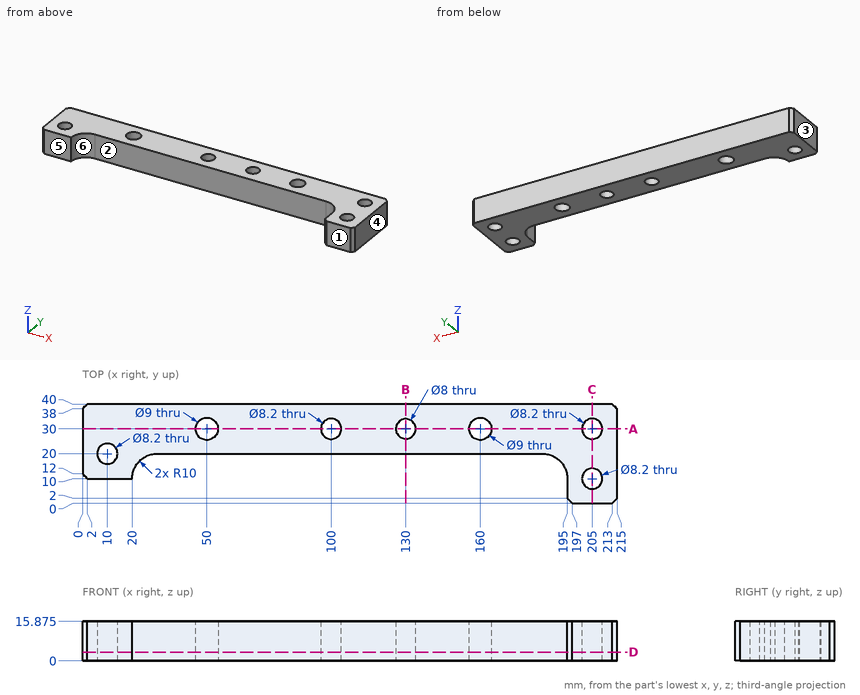
Study the drawing (mm; zero at the part's minimum x, y, z) and answer. A direction names the side the tool comes from. Coordinates: 2 decimals unless noted, no trailing zeros. Write each loop counter-clockwise with the first axis right and the second up, starting at its lowest first coordinate (ties: lowest second). Pieces come first, ordered by that corner, then holes. Notation, with made-up numbers: M -2.5,27.5 L 47.5,27.5 A18 ccw 47.5,33.5 Z; hole C 12.25,33.25 d11. An arc over 180 degrees is marked long. Use a Markdown table: item, result. Add a question column.
1. For a pull along X with two mould halves and no side action, classify the marked faces 3, 4, 5 and 6 as +X half, -X half, draft (parallel to the pull), parting line (faces both ways), or undercut.
2. Section D-D (z = 3.5) is taken. Count the separate pieces of the cut face and the enclosed holes in it, plus the area to 3 significant figures.
3. Section B-B (x = 130) is taken. Give the vertices of the cut face in (y, z) (3 decimals), plus the area to 4 significant figures.
4. Which of the six approach directions +Z, -Z, +X, -X, +Y, -Y give full straight-line access (tool end or side, diameter ignored) to the marked faces 1 and 2?
5. Straight lines are drawn through the part: line 1 along Y through (x, z) = (205, 6.5); line 2 along Y through (x, z) = (10, 6); line 3 along X through (y, z) = (29.5, 12). For each, find the intervals that lie inside material, in ascending order. Write a range as [from, to].
6. Section C-C (x = 205) is taken. Give the vertices of the cut face in (y, z) (3 decimals), plus the area to 3 significant figures.
7. Given P1, Ø8, axis at x = 50, y = 30, coming from the +Z side; P2, Ø2.5, axis at y = 5.5, z = 9, coming from the -X side; P3, Ø8, axis at x = 12, z = 7, coming from the -Y side, each flat-ended and moving along its own axis, determine where each tip first touches the part or whether it passes through.
8. Section A-A (y = 30) is taken. Give the vertices of the cut face in (x, z) (3 decimals).
Data:
| question | item | result |
|---|---|---|
| 1 | face 3 | -X half |
| 1 | face 4 | +X half |
| 1 | face 5 | draft |
| 1 | face 6 | undercut |
| 2 | separate pieces | 1 |
| 2 | enclosed holes | 7 |
| 2 | area | 4,540 mm2 |
| 3 | outline | M 20,0 L 26,0 L 26,15.875 L 20,15.875 Z; M 34,0 L 40,0 L 40,15.875 L 34,15.875 Z |
| 3 | area | 190.5 mm2 |
| 4 | face 1 | +Z, -Z, +X, -X, -Y |
| 4 | face 2 | +Z, -Z, -Y |
| 5 | line 1 | y = [0, 5.9], [14.1, 25.9], [34.1, 40] |
| 5 | line 2 | y = [10, 15.9], [24.1, 40] |
| 5 | line 3 | x = [0, 45.53], [54.47, 95.93], [104.07, 126.03], [133.97, 155.53], [164.47, 200.93], [209.07, 215] |
| 6 | outline | M 0,0 L 5.9,0 L 5.9,15.875 L 0,15.875 Z; M 14.1,0 L 25.9,0 L 25.9,15.875 L 14.1,15.875 Z; M 34.1,0 L 40,0 L 40,15.875 L 34.1,15.875 Z |
| 6 | area | 375 mm2 |
| 7 | P1 | passes through |
| 7 | P2 | stops at x = 195 |
| 7 | P3 | stops at y = 10 |
| 8 | outline | M 0,0 L 45.5,0 L 45.5,15.875 L 0,15.875 Z; M 54.5,0 L 95.9,0 L 95.9,15.875 L 54.5,15.875 Z; M 104.1,0 L 126,0 L 126,15.875 L 104.1,15.875 Z; M 134,0 L 155.5,0 L 155.5,15.875 L 134,15.875 Z; M 164.5,0 L 200.9,0 L 200.9,15.875 L 164.5,15.875 Z; M 209.1,0 L 215,0 L 215,15.875 L 209.1,15.875 Z |
